Design review of the part built by this model. Coordinates are the model's own, in mm. Face numbers are marked on the shaded views. Give positions to 0.01 mm unless a question says otherwise; leave off trailing zeros. Write each loop counter-clockwise with the first axis right and the second up, starting at its lowest first coordinate (ties: lowest second). Pieces come first, ordered by that corner, then holes. Notation, with made-up numbers: (78.5, 6.5) - (129.5, 6.5) arc R13 cw to (129.5, 22.5) - close; hole circle Ø1 at (-21.5, 42.25). An arc over 180 degrees is marked (long way). Use a Markdown table: item, result. Add a question column.
```python
from build123d import *

# Parameters (mm, degrees)
SKETCH_1_W          = 13
SKETCH_1_H          = 38
EXTRUDE_1_DEPTH     = 1
SKETCH_2_R          = 2
EXTRUDE_2_DEPTH     = 38
CUT_EXTRUDE_2_DEPTH = 10
SKETCH_4_R          = 2.5
CUT_EXTRUDE_3_DEPTH = 2


with BuildPart() as part:
    # 草图1 → 凸台-拉伸1 (new body)
    with BuildSketch(Plane.XY):
        Rectangle(SKETCH_1_W, SKETCH_1_H)
    extrude(amount=EXTRUDE_1_DEPTH)

    # 草图2 → 凸台-拉伸2 (add)
    with BuildSketch(Plane(origin=(0, 19, 0), x_dir=(1, 0, 0), z_dir=(0, 1, 0))):
        with BuildLine():
            Line((6.5, -1), (9, -1))
            ThreePointArc((9, -1), (10.767766953, 3.267766953), (6.5, 1.5))
            Line((6.5, 1.5), (6.5, -1))
        make_face()
        with Locations((9, 1.5)):
            Circle(SKETCH_2_R, mode=Mode.SUBTRACT)
    extrude(amount=-EXTRUDE_2_DEPTH)

    # 草图3 → 切除-拉伸2 (cut)
    with BuildSketch(Plane.XY.offset(1)):
        Polygon((5.480957084, 6.99044612), (5.442845313, 20.990394244), (12.442819375, 21.00945013), (12.480931146, 7.009502005), align=None)
        Polygon((5.442845313, -20.990394244), (12.442819375, -21.00945013), (12.480931146, -7.009502005), (5.480957084, -6.99044612), align=None)
    extrude(amount=-CUT_EXTRUDE_2_DEPTH, mode=Mode.SUBTRACT)

    # 草图4 → 切除-拉伸3 (cut)
    with BuildSketch(Plane(origin=(0, 0, 0), x_dir=(-1, 0, 0), z_dir=(0, 0, -1))):
        with Locations((1, 12.5)):
            Circle(SKETCH_4_R)
        with Locations((1, -12.5)):
            Circle(SKETCH_4_R)
    extrude(amount=-CUT_EXTRUDE_3_DEPTH, mode=Mode.SUBTRACT)


solid = part.part
```
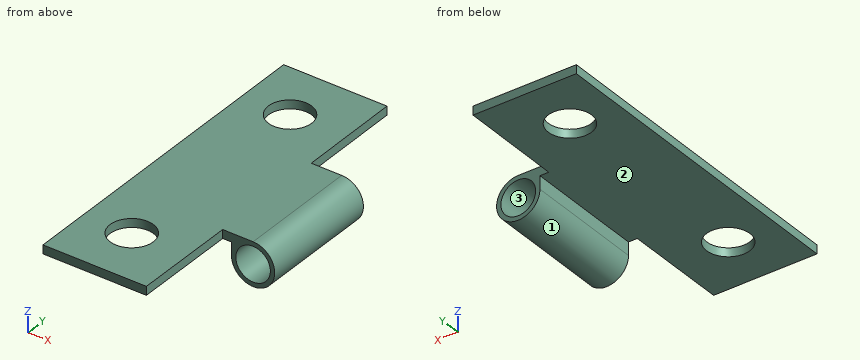
(1) Add section B-B (y = 14.5). State the section outline as (x, z) points, and give its area (3 significant figures).
(2) Add section A-A (x = -1). State the section outline as (y, z) points.
(3) Add section C-C (z = -0.35). State the section outline as (x, y) points.
(4) Mouldability with a two-part tool opening along X and no side actions: class the marked faces 1, 2 and 3 as +X half, -X half, draft (parallel to the pull), parting line (faces both ways), or undercut.
(5) Add section D-D (y = 6). State the section outline as (x, z) points.
(6) For line 1 along Y through (x, z) = (-1, 0.7); line 2 along X through (y, z) = (-1, -1.5); line 3 along Z through (x, y) = (9, -3), list the stretches that pass through material, from the lowest coordinate up.
(7) Insertion check: pin 1 (5 mm diameter, centred on x = -1, y = 6, fed in from -Z). The pin has a flat end and moves straight along its axis. Give the tip position at first contact, or say it passes through.
Answers follow:
| question | item | result |
|---|---|---|
| 1 | outline | (-6.5, 0) - (-2.5, 0) - (-2.5, 1) - (-6.5, 1) - close; (0.5, 0) - (5.46, 0) - (5.46, 1) - (0.5, 1) - close |
| 1 | area | 8.96 mm^2 |
| 2 | outline | (-19, 0) - (-15, 0) - (-15, 1) - (-19, 1) - close; (-10, 0) - (10, 0) - (10, 1) - (-10, 1) - close; (15, 0) - (19, 0) - (19, 1) - (15, 1) - close |
| 3 | outline | (6.5, -6.99) - (7.36, -7) - (7.36, 7) - (6.5, 6.99) - close; (10.64, -7) - (11.22, -7.01) - (11.22, 7.01) - (10.64, 7) - close |
| 4 | face 1 | parting line |
| 4 | face 2 | draft |
| 4 | face 3 | undercut |
| 5 | outline | (-6.5, 0) - (6.5, 0) - (6.5, -1.5) arc R2.5 ccw (long way) to (9, 1) - (-6.5, 1) - close; hole circle Ø4 at (9, -1.5) |
| 6 | line 1 | -19 to -15, -10 to 10, 15 to 19 |
| 6 | line 2 | 6.5 to 7, 11 to 11.5 |
| 6 | line 3 | -4 to -3.5, 0.5 to 1 |
| 7 | pin 1 | z = 0 |
